Work out the finished part from the listing and answer in its coordinate system (mm). Face numbers are marked on the shaded views. A direction names the side the tool comes from. Give positions to 0.01 mm unless a question says otherwise; leave off trailing zeros. Loops run counter-clockwise (first coordinate to the right, second up) from the corner with the lowest first, then second, coordinate; pieces in that order, holes last. Notation, with made-up numbers: M 50.25,9 L 69.25,9 A21 cw 69.25,39 Z; hole C -31,31 d8. An arc over 180 degrees is marked long. Use a Markdown table: item, result.
```python
from build123d import *

# Parameters (mm, degrees)
SKETCH1_W               = 20
SKETCH1_H               = 20
BOSS_EXTRUDE1_DEPTH     = 5
SKETCH2_W               = 20
SKETCH2_H               = 5
BOSS_EXTRUDE2_DEPTH     = 15
CUT_EXTRUDE1_DEPTH      = 21.615528128
CUT_EXTRUDE1_DEPTH_BACK = 21.615528128
SKETCH3_R               = 1.5
CUT_EXTRUDE2_DEPTH      = 27.925824036
CUT_EXTRUDE2_DEPTH_BACK = 27.925824036
SKETCH4_R               = 1.5
FILLET1_R               = 3


with BuildPart() as part:
    # Sketch1 → Boss-Extrude1 (new body)
    with BuildSketch(Plane(origin=(0, 0, 0), x_dir=(1, 0, 0), z_dir=(0, 1, 0))):
        Rectangle(SKETCH1_W, SKETCH1_H)
    extrude(amount=BOSS_EXTRUDE1_DEPTH)

    # Sketch2 → Boss-Extrude2 (add)
    with BuildSketch(Plane(origin=(0, 5, 0), x_dir=(1, 0, 0), z_dir=(0, 1, 0))):
        with Locations((0, 7.5)):
            Rectangle(SKETCH2_W, SKETCH2_H)
    extrude(amount=BOSS_EXTRUDE2_DEPTH)

    # Sketch3 → Cut-Extrude1 (cut, two sides: drawn at the far end of the back side and taken through both)
    with BuildSketch(Plane(origin=(0, 5, 0), x_dir=(1, 0, 0), z_dir=(0, 1, 0)).offset(-CUT_EXTRUDE1_DEPTH_BACK)):
        with Locations(Location((-5, -3, 0), (0, 0, 270))):
            Circle(SKETCH3_R)
        with Locations(Location((5, -3, 0), (0, 0, 90))):
            Circle(SKETCH3_R)
    extrude(amount=CUT_EXTRUDE1_DEPTH + CUT_EXTRUDE1_DEPTH_BACK, mode=Mode.SUBTRACT)

    # Sketch4 → Cut-Extrude2 (cut, two sides: drawn at the far end of the back side and taken through both)
    with BuildSketch(Plane.XY.offset(-5).offset(-CUT_EXTRUDE2_DEPTH_BACK)):
        with Locations((-5, 13)):
            Circle(SKETCH4_R)
        with Locations(Location((5, 13, 0), (0, 0, 180))):
            Circle(SKETCH4_R)
    extrude(amount=CUT_EXTRUDE2_DEPTH + CUT_EXTRUDE2_DEPTH_BACK, mode=Mode.SUBTRACT)

    # Fillet1
    fillet1_edges = [part.edges().sort_by_distance(p)[0] for p in [
        (0, 5, -5),
    ]]
    fillet(fillet1_edges, radius=FILLET1_R)


solid = part.part
```
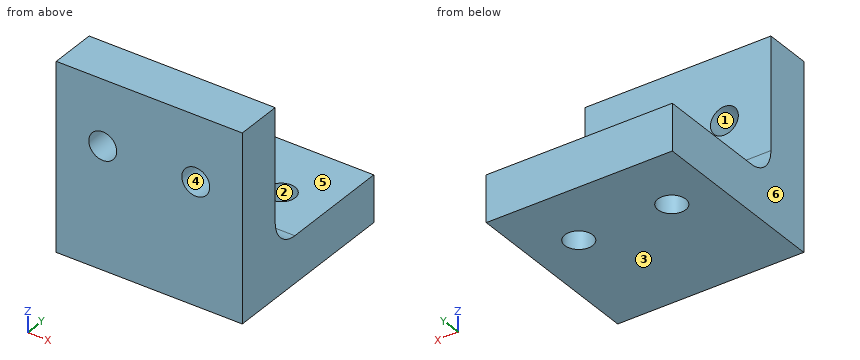
(1) A cutting plane is placed at C-C (y = 13). Write down the section's boundary in (x, z), and give its area (3 significant figures).
Entries:
| item | result |
|---|---|
| outline | M -10,-10 L -6.5,-10 L -6.5,-5 L -10,-5 Z; M -3.5,-10 L 3.5,-10 L 3.5,-5 L -3.5,-5 Z; M 6.5,-10 L 10,-10 L 10,-5 L 6.5,-5 Z |
| area | 70.0 mm² |
(2) The mould has two halves that part along Z. Classify the marked faces 1, 2, 3 and 4: released by +Z, released by -Z, zero draft, split by the parting line, or undercut.
Entries:
| item | result |
|---|---|
| face 1 | undercut |
| face 2 | zero draft |
| face 3 | released by -Z |
| face 4 | undercut |
(3) Consider probe 1 along Y at (x, z) = (5, -6.15); probe 2 along Y at (x, z) = (5, -2); probe 3 along Z at (x, y) = (-5, 3.3). Determine where each line is inside the solid, lowest interval first. Write a range as [from, to].
Entries:
| item | result |
|---|---|
| probe 1 | y = [0, 11.5], [14.5, 20] |
| probe 2 | y = [0, 5] |
| probe 3 | z = [-10, 1.5], [4.5, 10] |
(4) A cutting plane is placed at B-B (x = 5). Write down the section's boundary in (y, z).
Entries:
| item | result |
|---|---|
| outline | M 0,-10 L 11.5,-10 L 11.5,-5 L 8,-5 A3 cw 5,-2 L 5,1.5 L 0,1.5 Z; M 0,4.5 L 5,4.5 L 5,10 L 0,10 Z; M 14.5,-10 L 20,-10 L 20,-5 L 14.5,-5 Z |
(5) A cutting plane is placed at D-D (x = -1.5). Write down the section's boundary in (y, z).
Entries:
| item | result |
|---|---|
| outline | M 0,-10 L 20,-10 L 20,-5 L 8,-5 A3 cw 5,-2 L 5,10 L 0,10 Z |
(6) A cutting plane is placed at A-A (z = 3). Write down the section's boundary in (x, y), and give its area (3 significant figures).
Entries:
| item | result |
|---|---|
| outline | M -10,0 L -6.5,0 L -6.5,5 L -10,5 Z; M -3.5,0 L 3.5,0 L 3.5,5 L -3.5,5 Z; M 6.5,0 L 10,0 L 10,5 L 6.5,5 Z |
| area | 70.0 mm² |
(7) Which of the six approach directions +Z, -Z, +X, -X, +Y, -Y give full straight-line access (tool end or side, diameter ignored) to the marked faces 5 and 6?
Entries:
| item | result |
|---|---|
| face 5 | +Z, +X, -X, +Y |
| face 6 | +Z, -Z, -X, +Y, -Y |
(8) Given P1, Ø3.5, axis at x = 5, z = 3, coming from the +Y side; P2, Ø2, axis at x = 4, z = -2, coming from the -Y side; P3, Ø1.8, axis at x = -5, z = 3, coming from the -Y side; P4, Ø6, axis at x = -3, y = 16, coming from the +Z side, each flat-ended and moving along its own axis, determine where each tip first touches the part or whether it passes through.
Entries:
| item | result |
|---|---|
| P1 | stops at y = 5 |
| P2 | stops at y = 0 |
| P3 | passes through |
| P4 | stops at z = -5 |
